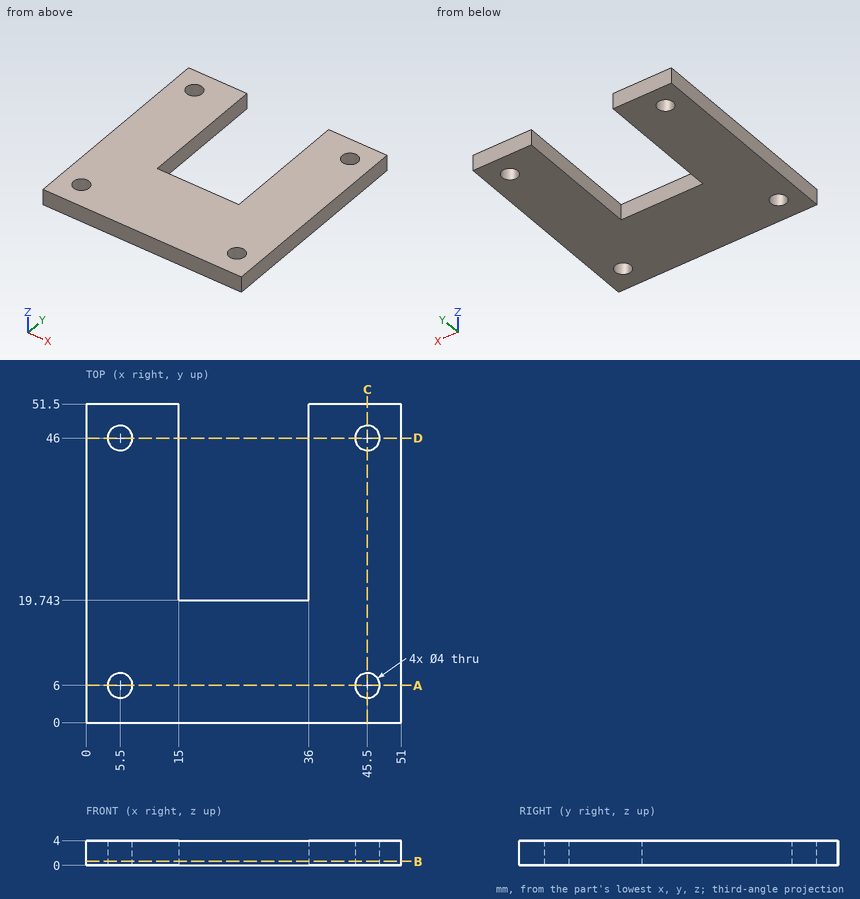
Check sheet for the drawn part. Datum: minimum x, y, z corner. Units: mm. Give positions to 0.01 mm unless a question says otherwise; leave off trailing zeros. Order: outer loops, then holes, each group sorted by start corner. A loop starts at its lowest first (then second) coordinate and runs counter-clockwise, first axis right, second up. Notation, with made-up numbers: (35, -5) - (70, -5) arc R33 ccw to (70, 32) - close; hole circle Ø1 at (15.25, 44.5). An arc over 180 degrees is marked (long way). Answer in a Markdown table with one row per item. Add a question column.
Q1. Cross-section at B-B, the plane z = 0.65. Enter the section's corners in (x, y).
Q2. Gauge pin test, flat ends, axial feed: pin 1 (3.5 mm diameter, centred on x = 5.5, y = 6, fed in from +Z); pin 2 (1 mm diameter, centred on x = 22, z = 2.5, fed in from +Y). Record the tip position at first contact, or that the pin passes through.
Q3. Material ranges on probe 1 along Y at (x, z) = (45.5, 1.6); probe 2 along X at (y, z) = (40.5, 3.45); probe 3 along X at (y, z) = (44.5, 3.1), recorded low to high. Write a range as from..to.
Q4. Cross-section at A-A, the plane y = 6. Enter the section's corners in (x, z), then the cut area to 3 significant figures.
Q5. Cross-section at D-D, the plane y = 46. Enter the section's corners in (x, z).
Q6. Cross-section at C-C, the plane x = 45.5. Enter the section's corners in (y, z).
Check values:
| question | item | result |
|---|---|---|
| 1 | outline | (0, 0) - (51, 0) - (51, 51.5) - (36, 51.5) - (36, 19.74) - (15, 19.74) - (15, 51.5) - (0, 51.5) - close; hole circle Ø4 at (5.5, 6); hole circle Ø4 at (5.5, 46); hole circle Ø4 at (45.5, 6); hole circle Ø4 at (45.5, 46) |
| 2 | pin 1 | passes through |
| 2 | pin 2 | stops at y = 19.74 |
| 3 | probe 1 | y = 0..4, 8..44, 48..51.5 |
| 3 | probe 2 | x = 0..15, 36..51 |
| 3 | probe 3 | x = 0..4.18, 6.82..15, 36..44.18, 46.82..51 |
| 4 | outline | (0, 0) - (3.5, 0) - (3.5, 4) - (0, 4) - close; (7.5, 0) - (43.5, 0) - (43.5, 4) - (7.5, 4) - close; (47.5, 0) - (51, 0) - (51, 4) - (47.5, 4) - close |
| 4 | area | 172 mm^2 |
| 5 | outline | (0, 0) - (3.5, 0) - (3.5, 4) - (0, 4) - close; (7.5, 0) - (15, 0) - (15, 4) - (7.5, 4) - close; (36, 0) - (43.5, 0) - (43.5, 4) - (36, 4) - close; (47.5, 0) - (51, 0) - (51, 4) - (47.5, 4) - close |
| 6 | outline | (0, 0) - (4, 0) - (4, 4) - (0, 4) - close; (8, 0) - (44, 0) - (44, 4) - (8, 4) - close; (48, 0) - (51.5, 0) - (51.5, 4) - (48, 4) - close |
